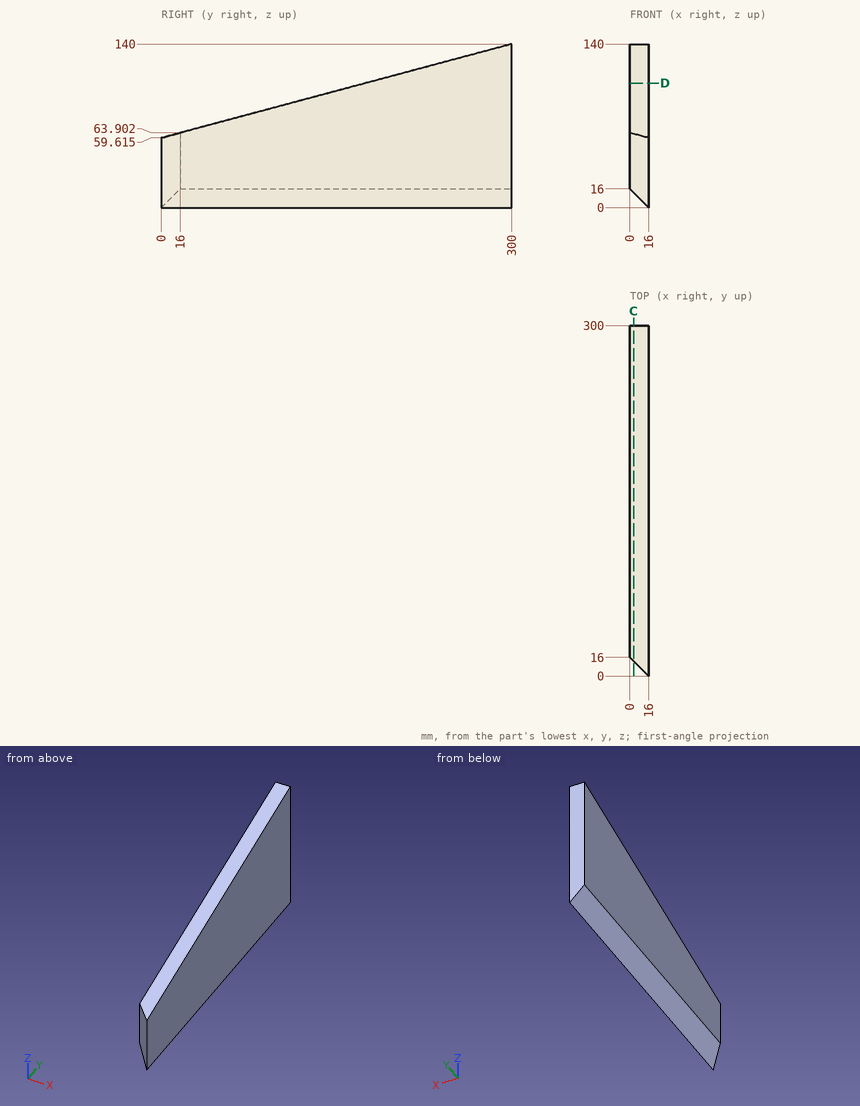
Design review of the part shown in the three views and the two pictorial views. Dimensions are in mm from the part's minimum x, y and z. Coordinates: 2 decimals unless noted, no trailing zeros. Write each loop counter-clockwise with the first axis right and the second up, starting at its lowest first coordinate (ties: lowest second). Pieces come first, ordered by that corner, then holes.
1) To check wall thickness, follow probe 1 along Z at (x, y) = (0.5, 153.5) (1 decimal); probe 2 along Z at (x, y) = (8.5, 273.5); probe 3 along X at (y, z) = (241.5, 15.5). State the ranges of each line that lie inside material, in increasing order.
2) We need section D-D on z = 106.5. State the section outline as (x, y) points.
3) Clearance check with flat-ended pins moving along their axes: pin 1 Ø1.5 at (x, y) = (7, 196) entering from +Z (1 decimal); pin 2 Ø1 at (x, z) = (5.5, 25.5) entering from -Y; pin 3 Ø3 at (x, y) = (7.5, 79.5) entering from -Z. State where each tip first meets the part, or that it passes through.
4) We need section C-C on x = 3.25. State the section outline as (y, z) points.
Answer list:
1. probe 1: z = 15.5 to 100.7
1. probe 2: z = 7.5 to 132.9
1. probe 3: x = 0.5 to 16
2. outline: (0, 174.98) - (16, 174.98) - (16, 300) - (0, 300) - close
3. pin 1: stops at z = 112.3
3. pin 2: stops at y = 10
3. pin 3: stops at z = 7
4. outline: (12.75, 12.75) - (300, 12.75) - (300, 140) - (12.75, 63.03) - close
